For this review, take the finished solid that the model builds, in its own axes (mm). Round coordinates to 2 decimals unless told otherwise and drop trailing zeros. Write each loop counter-clockwise with the first axis right and the second up, starting at its lowest first coordinate (ties: lowest second). Pieces come first, ordered by that corner, then holes. Notation, with made-up numbers: M 5.5,45.5 L 64.5,45.5 A29 cw 64.5,84.5 Z; hole C -35,78 d5. An arc over 180 degrees is marked long. Answer in a Markdown table with one row per item.
```python
from build123d import *

# Parameters (mm, degrees)
SKETCH1_R           = 12.5
BOSS_EXTRUDE1_DEPTH = 17.6
SKETCH2_R           = 5.5
CUT_EXTRUDE1_DEPTH  = 50.8
SKETCH3_R           = 8
CUT_EXTRUDE3_DEPTH  = 15.6
BOSS_EXTRUDE2_DEPTH = 17.6
SKETCH6_R           = 8
SKETCH6_R_2         = 5.5
CUT_EXTRUDE5_DEPTH  = 14.425


with BuildPart() as part:
    # Sketch1 → Boss-Extrude1 (new body)
    with BuildSketch(Plane(origin=(0, 0, 0), x_dir=(1, 0, 0), z_dir=(0, 1, 0))):
        with Locations(Location((0, 0, 0), (0, 0, 270))):
            Circle(SKETCH1_R)
    extrude(amount=BOSS_EXTRUDE1_DEPTH)

    # Sketch2 → Cut-Extrude1 (cut)
    with BuildSketch(Plane(origin=(0, 17.6, 0), x_dir=(1, 0, 0), z_dir=(0, 1, 0))):
        with Locations(Location((0, 0, 0), (0, 0, 270))):
            Circle(SKETCH2_R)
    extrude(amount=-CUT_EXTRUDE1_DEPTH, mode=Mode.SUBTRACT)

    # Sketch3 → Cut-Extrude3 (cut)
    with BuildSketch(Plane(origin=(0, 17.6, 0), x_dir=(1, 0, 0), z_dir=(0, 1, 0))):
        with Locations(Location((0, 0, 0), (0, 0, 270))):
            Circle(SKETCH3_R)
    extrude(amount=-CUT_EXTRUDE3_DEPTH, mode=Mode.SUBTRACT)

    # Sketch5 → Boss-Extrude2 (add, through all)
    with BuildSketch(Plane(origin=(0, 17.6, 0), x_dir=(1, 0, 0), z_dir=(0, 1, 0))):
        with BuildLine():
            ThreePointArc((12.5, 0), (12.085103338, -3.193787298), (10.867955631, -6.175559927))
            Line((10.867955631, -6.175559927), (24.985285623, 18.668586645))
            Line((24.985285623, 18.668586645), (8.74807309, 27.895149805))
            Line((8.74807309, 27.895149805), (0, 12.5))
            ThreePointArc((0, 12.5), (8.838834765, 8.838834765), (12.5, 0))
        make_face()
    extrude(amount=-BOSS_EXTRUDE2_DEPTH)

    # Sketch6 → Cut-Extrude5 (cut)
    with BuildSketch(Plane.XZ):
        with BuildLine():
            Line((24.985285623, -18.668586645), (10.867955631, 6.175559927))
            ThreePointArc((10.867955631, 6.175559927), (-10.803807178, 6.287109865), (0, -12.5))
            Line((0, -12.5), (8.74807309, -27.895149805))
            Line((8.74807309, -27.895149805), (24.985285623, -18.668586645))
        make_face()
        with Locations(Location((0, 0, 0), (0, 0, 90))):
            Circle(SKETCH6_R, mode=Mode.SUBTRACT)
        with Locations(Location((0, 0, 0), (0, 0, 90))):
            Circle(SKETCH6_R)
        Circle(SKETCH6_R_2, mode=Mode.SUBTRACT)
    extrude(amount=-CUT_EXTRUDE5_DEPTH, mode=Mode.SUBTRACT)


solid = part.part
```
Q1. Take a section at D-D (x = 23.5). State the section outline as (y, z) points (3 decimals).
Found:
| item | result |
|---|---|
| outline | M 14.425,-19.513 L 17.6,-19.513 L 17.6,-16.055 L 14.425,-16.055 Z |
Q2. Take a section at C-C (x = -3). State the section outline as (y, z) points (3 decimals), then the cut area to 3 significant figures.
Found:
| item | result |
|---|---|
| outline | M 14.425,-12.135 L 17.6,-12.135 L 17.6,-7.416 L 14.425,-7.416 Z; M 14.425,7.416 L 17.6,7.416 L 17.6,12.135 L 14.425,12.135 Z |
| area | 30.0 mm² |
Q3. Mouldability with a two-part tool opening along Z and no side actions: class faces 1 (the face through (16.98, 16.035, -23.217)), 2 (the face through (7, 17.6, -8)), 3 (the face through (-7.81, 16.03, -1.73)), 4 (the face through (17.828, 16.035, -6.073)) as +Z half, -Z half, draft (parallel to the pull), parting line (faces both ways), or undercut.
Found:
| item | result |
|---|---|
| face 1 | -Z half |
| face 2 | draft |
| face 3 | undercut |
| face 4 | +Z half |
Q4. Take a section at B-B (y = 16.05). State the section outline as (x, z) points, then the cut area to 3 significant figures.
Found:
| item | result |
|---|---|
| outline | M 0,-12.5 L 8.75,-27.9 L 24.99,-18.67 L 10.87,6.18 A12.5 ccw long Z; hole C 0,0 d16 |
| area | 627 mm² |
Q5. Take a section at A-A (z = 1.5). State the section outline as (x, y) points (3 decimals), then the cut area to 3 significant figures.
Found:
| item | result |
|---|---|
| outline | M -12.41,14.425 L -7.858,14.425 L -7.858,17.6 L -12.41,17.6 Z; M 7.858,14.425 L 13.525,14.425 L 13.525,17.6 L 7.858,17.6 Z |
| area | 32.4 mm² |
Q6. For probe 1 along X at (y, z) = (14.8, 1.5); probe 2 along X at (y, z) = (15.45, 0); probe 3 along Z at (x, y) = (-3, 14.8), list the stretches that pass through material, from the lowest coordinate up.
Found:
| item | result |
|---|---|
| probe 1 | -12.41 to -7.86, 7.86 to 13.52 |
| probe 2 | -12.5 to -8, 8 to 14.38 |
| probe 3 | -12.13 to -7.42, 7.42 to 12.13 |
Q7. Insertion check: P1, Ø1, axis at x = 17, y = 16, coming from the -Z side; P2, Ø1, axis at x = -8, y = 15.5, coming from the -Z side; P3, Ø1, axis at x = -5.5, y = 15.5, coming from the -Z side. Each pin has a flat end and moves straight along its axis. Give the tip position at first contact, or say it passes through.
Found:
| item | result |
|---|---|
| P1 | z = -23.49 |
| P2 | z = -10 |
| P3 | z = -11.46 |
